Here's how the part is built. I have some questions about the finished solid (model axes, mm). Round coordinates to 2 decimals unless told otherwise and drop trailing zeros. Order: outer loops, then holes, each group sorted by start corner. A loop starts at its lowest first (then second) coordinate and runs counter-clockwise, first axis right, second up. Notation, with made-up numbers: (22, 20) -> (28, 20) arc R21 cw to (28, 42) -> close; hole circle Ø6 at (-20.75, 20). An arc over 180 degrees is marked (long way). Use a Markdown table: item, result. Add a question column.
(1) I'm going to push a flat-ended pin straight in: P1, Ø3, axis at y = 6.5, z = 1.5, coming from the +X side. Where does the tip first touch, or does it pass through?
(2) I want a section at A-A, the plane y = 4. Please give me the cut outline in (x, z), then the cut area to 3 significant figures.
(3) If I drill on probe 1 along Z at (x, y) = (113, 1.25); probe 2 along Z at (x, y) = (87, 6); probe 3 along X at (y, z) = (7.5, 61.5), over which ranges is the centre line in solid material (lowest first)?
from build123d import *

# Parameters (mm, degrees)
BOSS_EXTRUDE1_DEPTH = 7.62
FILLET1_R           = 2.54
SCALE1_SCALE        = 1.5


with BuildPart() as part:
    # Sketch1 → Boss-Extrude1 (new body)
    with BuildSketch(Plane(origin=(0, 0, 0), x_dir=(1, 0, 0), z_dir=(0, 1, 0))):
        with BuildLine():
            Line((15.948005464, 0), (212.651994536, 0))
            ThreePointArc((212.651994536, 0), (221.220851626, -4.701035979), (221.860081653, -14.453801539))
            Line((221.860081653, -14.453801539), (192.841756086, -76.683801539))
            ThreePointArc((192.841756086, -76.683801539), (189.09263299, -80.958857089), (183.63366897, -82.55))
            Line((183.63366897, -82.55), (44.96633103, -82.55))
            ThreePointArc((44.96633103, -82.55), (39.50736701, -80.958857089), (35.758243914, -76.683801539))
            Line((35.758243914, -76.683801539), (6.739918347, -14.453801539))
            ThreePointArc((6.739918347, -14.453801539), (7.379148374, -4.701035979), (15.948005464, 0))
        make_face()
    extrude(amount=BOSS_EXTRUDE1_DEPTH)

    # Fillet1
    fillet1_edges = [part.edges().sort_by_distance(p)[0] for p in [
        (7.379148374, 7.62, 4.701035979),
        (114.3, 0, 0),
        (221.220851626, 0, 4.701035979),
        (21.249081131, 7.62, 45.568801539),
        (39.50736701, 7.62, 80.958857089),
        (114.3, 7.62, 82.55),
        (189.09263299, 7.62, 80.958857089),
        (207.350918869, 7.62, 45.568801539),
        (221.220851626, 7.62, 4.701035979),
        (114.3, 7.62, 0),
        (207.350918869, 0, 45.568801539),
        (189.09263299, 0, 80.958857089),
        (114.3, 0, 82.55),
        (39.50736701, 0, 80.958857089),
        (21.249081131, 0, 45.568801539),
        (7.379148374, 0, 4.701035979),
    ]]
    fillet(fillet1_edges, radius=FILLET1_R)


with BuildPart() as part_1:
    # Scale1: scaled about (114.3, 3.81, 38.735119428)
    add(part.part.scale(SCALE1_SCALE).moved(Location((-57.15, -1.905, -19.367559714))))


solid = part_1.part
Taken from the geometry:
| question | item | result |
|---|---|---|
| 1 | P1 | stops at x = 276.46 |
| 2 | outline | (-47.04, 2.31) arc R15.24 ccw to (-33.23, -19.37) -> (261.83, -19.37) arc R15.24 ccw to (275.64, 2.31) -> (232.11, 95.66) arc R15.24 ccw to (218.3, 104.46) -> (10.3, 104.46) arc R15.24 ccw to (-3.51, 95.66) -> close |
| 2 | area | 35,000 mm2 |
| 3 | probe 1 | z = -19.31 to 104.4 |
| 3 | probe 2 | z = -19.36 to 104.45 |
| 3 | probe 3 | x = -18.95 to 247.55 |
